Could you check a few things on this drawing? It's one solid part, dimensions in mm from its lowest x, y, z. Give positions to 0.01 mm unless a question says otherwise; leave off trailing zeros. Loops run counter-clockwise (first coordinate to the right, second up) from the corner with the lowest first, then second, coordinate; pieces in that order, holes last. Notation, with made-up numbers: (64.25, 47) -> (120.25, 47) arc R15 ccw to (120.25, 74) -> close; hole circle Ø8 at (8.25, 26). An arc over 180 degrees is marked (long way). One line per question, with ' | ' between items.
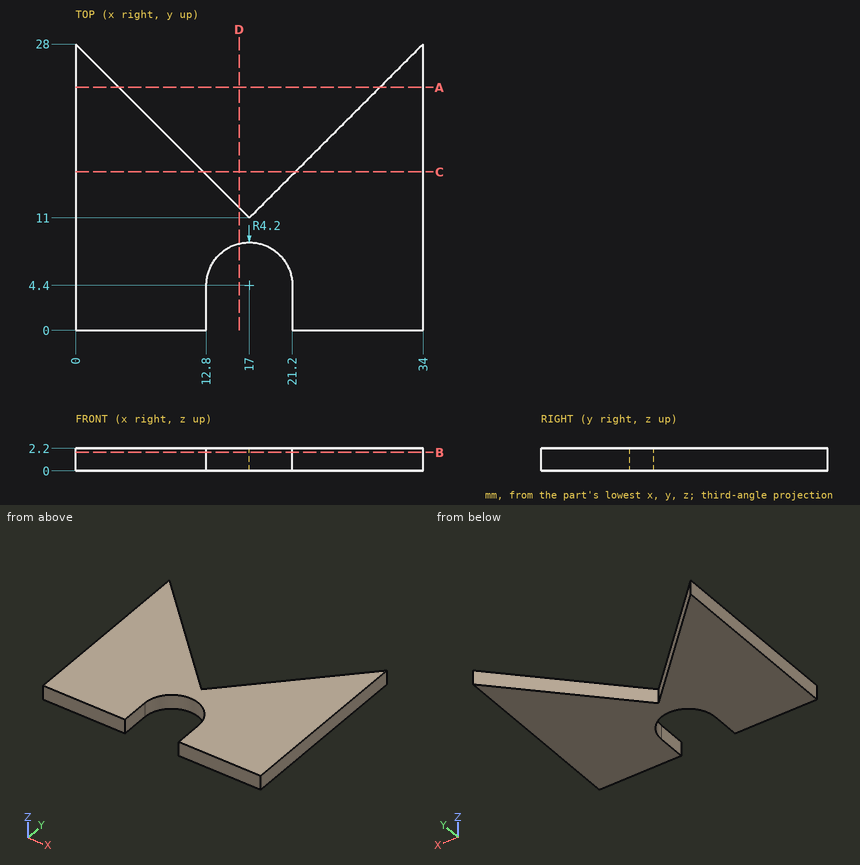
Q1. For pin 1 Ø5 at (x, y) = (23.5, 23) entering from +Z, with a flat end and sliding along its axis, tell me the tip position at first contact or that it passes through.
Entries:
pin 1: through
Q2. If I drill on probe 1 along X at (y, z) = (2.75, 0.1); probe 2 along X at (y, z) = (11.75, 1.6); probe 3 along Y at (x, z) = (28.5, 0.6), over which ranges is the centre line in solid material (lowest first)? Write a range as from..to.
Entries:
probe 1: 0..12.8, 21.2..34 | probe 2: 0..16.25, 17.75..34 | probe 3: 0..22.5
Q3. If we section it at A-A (y = 23.75): Write out the boundary of the cut face in (x, z), plus the area to 3 significant figures.
Entries:
outline: (0, 0) -> (4.25, 0) -> (4.25, 2.2) -> (0, 2.2) -> close; (29.75, 0) -> (34, 0) -> (34, 2.2) -> (29.75, 2.2) -> close | area: 18.7 mm²
Q4. If we section it at D-D (x = 16): Write out the boundary of the cut face in (y, z), plus the area to 3 significant figures.
Entries:
outline: (8.48, 0) -> (12, 0) -> (12, 2.2) -> (8.48, 2.2) -> close | area: 7.75 mm²
Q5. If we section it at B-B (z = 1.8): Write out the boundary of the cut face in (x, y), plus the area to 3 significant figures.
Entries:
outline: (0, 0) -> (12.8, 0) -> (12.8, 4.4) arc R4.2 cw to (21.2, 4.4) -> (21.2, 0) -> (34, 0) -> (34, 28) -> (17, 11) -> (0, 28) -> close | area: 598 mm²
Q6. If we section it at C-C (y = 15.5): Write out the boundary of the cut face in (x, z).
Entries:
outline: (0, 0) -> (12.5, 0) -> (12.5, 2.2) -> (0, 2.2) -> close; (21.5, 0) -> (34, 0) -> (34, 2.2) -> (21.5, 2.2) -> close
